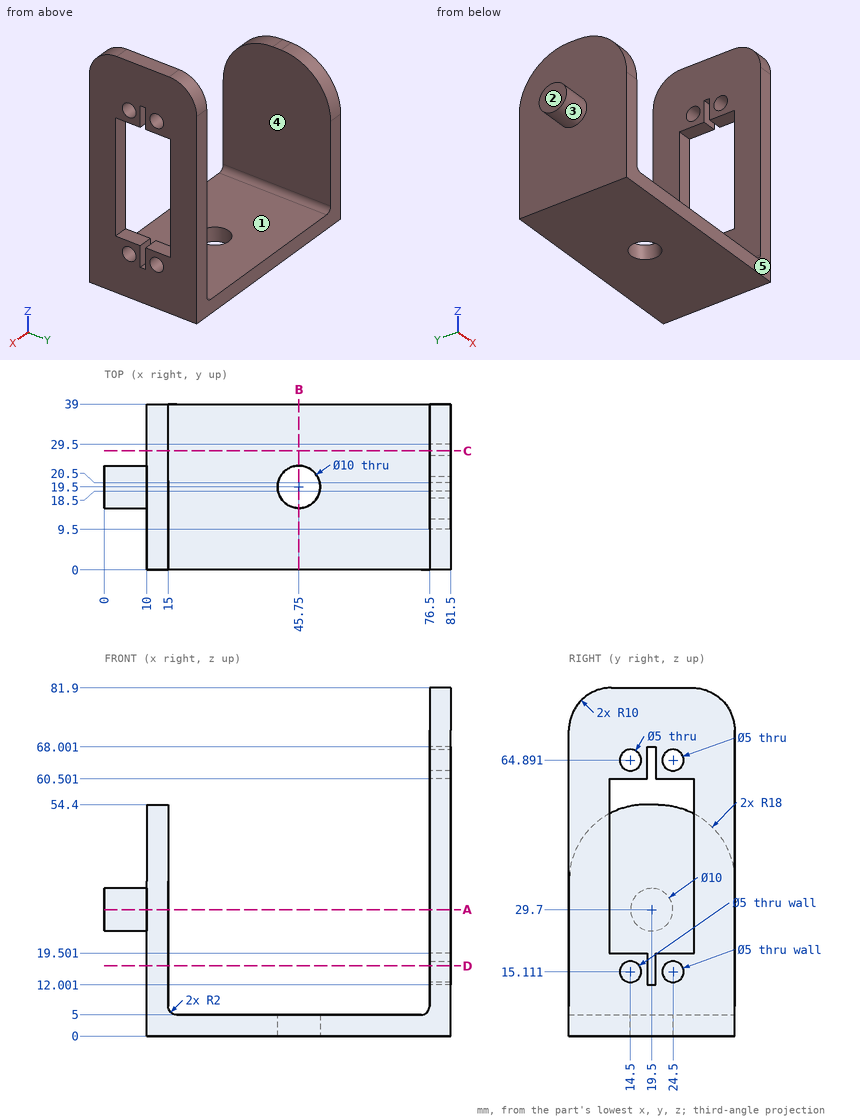
Can you work these out from the drawing? Everything is in mm from the part's minimum corner. A direction names the side the tool comes from. Coordinates: 2 decimals unless noted, no trailing zeros. Loops run counter-clockwise (first coordinate to the right, second up) from the corner with the lowest first, then second, coordinate; pieces in that order, holes last.
1) Which directions (+Z, -Z, +X, -X, +Y, -Y) give clear straight access to the entire face, cutting with the end or side of a thin tool? Please do the marked faces 4 and 5.
Reported:
face 4: +Z, +Y, -Y
face 5: +Z, -Z, +X, -X, -Y
2) Will these pins go through, and if not, where does the flat tip stop? pin 1 Ø6 at (x, y) = (45.75, 19.5) entering from +Z; pin 2 Ø4.5 at (y, z) = (14.5, 15.111) entering from +X; pin 3 Ø8 at (y, z) = (31, 20.5) entering from -X; pin 4 Ø3.5 at (x, y) = (12, 19.5) entering from +Z.
Reported:
pin 1: passes through
pin 2: stops at x = 15
pin 3: stops at x = 10
pin 4: stops at z = 54.4
3) Imagine slicing it at D-D (z = 16.5). List the corners of the cut face in (x, y) for me, and give its area (3 significant figures).
Reported:
outline: (10, 0) - (15, 0) - (15, 39) - (10, 39) - close; (76.5, 0) - (81.5, 0) - (81.5, 12.42) - (76.5, 12.42) - close; (76.5, 16.58) - (81.5, 16.58) - (81.5, 18.5) - (76.5, 18.5) - close; (76.5, 20.5) - (81.5, 20.5) - (81.5, 22.42) - (76.5, 22.42) - close; (76.5, 26.58) - (81.5, 26.58) - (81.5, 39) - (76.5, 39) - close
area: 338 mm2
4) Please list where these lines run through material, in increasing order: line 1 along X through (y, z) = (19.5, 2.5); line 2 along X through (y, z) = (32, 17); line 3 along Z through (x, y) = (78, 14).
Reported:
line 1: x = 10 to 40.75, 50.75 to 81.5
line 2: x = 10 to 15, 76.5 to 81.5
line 3: z = 0 to 12.66, 17.56 to 19.5, 60.5 to 62.44, 67.34 to 81.9
5) Thinking about a two-plate mould opening in X: for the marked faces 1, 2 and 3, which applies, released by +X, released by -X, zero draft, split by the parting line, or undercut?
Reported:
face 1: undercut
face 2: released by -X
face 3: zero draft
6) Imagine slicing it at C-C (y = 28). List the corners of the cut face in (x, z) for me.
Reported:
outline: (10, 0) - (81.5, 0) - (81.5, 19.5) - (76.5, 19.5) - (76.5, 7) arc R2 cw to (74.5, 5) - (17, 5) arc R2 cw to (15, 7) - (15, 52.98) - (10, 52.98) - close; (76.5, 60.5) - (81.5, 60.5) - (81.5, 81.9) - (76.5, 81.9) - close
7) Imagine slicing it at B-B (x = 45.75). List the corners of the cut face in (y, z) for me, and give its area (3 significant figures).
Reported:
outline: (0, 0) - (14.5, 0) - (14.5, 5) - (0, 5) - close; (24.5, 0) - (39, 0) - (39, 5) - (24.5, 5) - close
area: 145 mm2
8) Imagine slicing it at A-A (z = 29.7). List the corners of the cut face in (x, y) for me.
Reported:
outline: (0, 14.5) - (10, 14.5) - (10, 0) - (15, 0) - (15, 39) - (10, 39) - (10, 24.5) - (0, 24.5) - close; (76.5, 0) - (81.5, 0) - (81.5, 9.5) - (76.5, 9.5) - close; (76.5, 29.5) - (81.5, 29.5) - (81.5, 39) - (76.5, 39) - close
